Geometry: final body of the model. Coordinates: model frame, mm. Face numbers are marked on the shaded views. A direction names the side the tool comes from. Give positions to 0.01 mm unless a question says otherwise; leave off trailing zeros. Loops run counter-clockwise (first coordinate to the right, second up) from the corner with the lowest first, then second, coordinate; pieces in that order, holes last. Notation, with made-up numbers: (47, 11) - (105, 11) arc R22 cw to (105, 39) - close; hole circle Ø1 at (37.25, 12). An arc over 180 degrees is marked (long way). Answer in a Markdown table with one row per item.
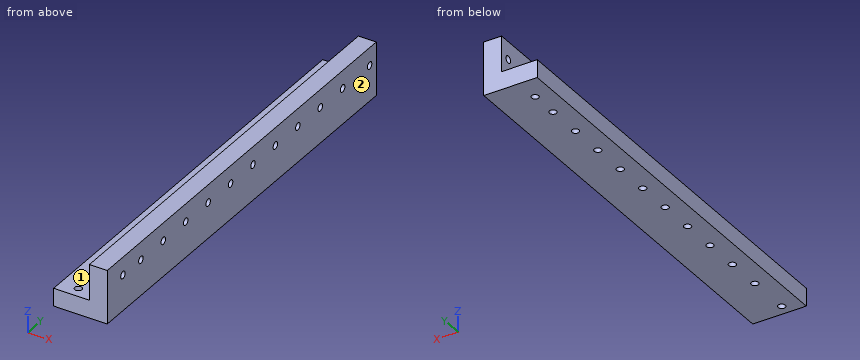
from build123d import *

# Parameters (mm, degrees)
BOSS_EXTRUDE1_DEPTH = 120
SKETCH2_R           = 1
CUT_EXTRUDE3_DEPTH  = 120
SKETCH4_R           = 1
CUT_EXTRUDE4_DEPTH  = 120
SKETCH5_R           = 1
CUT_EXTRUDE5_DEPTH  = 120
SKETCH6_R           = 1
CUT_EXTRUDE6_DEPTH  = 120
SKETCH8_R           = 1
CUT_EXTRUDE7_DEPTH  = 120
SKETCH9_R           = 1
CUT_EXTRUDE8_DEPTH  = 120


with BuildPart() as part:
    # Sketch1 → Boss-Extrude1 (new body)
    with BuildSketch(Plane(origin=(0, 0, 0), x_dir=(1, 0, 0), z_dir=(0, 1, 0))):
        Polygon((-19.661478752, 6.607142857), (-4.661478752, 6.607142857), (-4.661478752, -8.392857143), (-9.661478752, -8.392857143), (-9.661478752, 1.607142857), (-19.661478752, 1.607142857), align=None)
    extrude(amount=BOSS_EXTRUDE1_DEPTH)

    # Sketch2 → Cut-Extrude3 (cut)
    with BuildSketch(Plane(origin=(-4.661478752, 0, 0), x_dir=(0, 0, -1), z_dir=(1, 0, 0))):
        with Locations((-3.392857143, 117)):
            Circle(SKETCH2_R)
    extrude(amount=-CUT_EXTRUDE3_DEPTH, mode=Mode.SUBTRACT)

    # Sketch4 → Cut-Extrude4 (cut)
    with BuildSketch(Plane(origin=(0, 0, -6.607142857), x_dir=(-1, 0, 0), z_dir=(0, 0, -1))):
        with Locations((14.661478752, 113)):
            Circle(SKETCH4_R)
    extrude(amount=-CUT_EXTRUDE4_DEPTH, mode=Mode.SUBTRACT)

    # Sketch5 → Cut-Extrude5 (cut)
    with BuildSketch(Plane(origin=(-4.661478752, 0, 0), x_dir=(0, 0, -1), z_dir=(1, 0, 0))):
        with Locations((-3.392857143, 7)):
            Circle(SKETCH5_R)
    extrude(amount=-CUT_EXTRUDE5_DEPTH, mode=Mode.SUBTRACT)

    # Sketch6 → Cut-Extrude6 (cut)
    with BuildSketch(Plane(origin=(0, 0, -6.607142857), x_dir=(-1, 0, 0), z_dir=(0, 0, -1))):
        with Locations((14.661478752, 3)):
            Circle(SKETCH6_R)
    extrude(amount=-CUT_EXTRUDE6_DEPTH, mode=Mode.SUBTRACT)

    # Sketch8 → Cut-Extrude7 (cut)
    with BuildSketch(Plane(origin=(-4.661478752, 0, 0), x_dir=(0, 0, -1), z_dir=(1, 0, 0))):
        with Locations((-3.392857143, 105)):
            Circle(SKETCH8_R)
        with Locations((-3.392857143, 95)):
            Circle(SKETCH8_R)
        with Locations((-3.392857143, 85)):
            Circle(SKETCH8_R)
        with Locations((-3.392857143, 75)):
            Circle(SKETCH8_R)
        with Locations((-3.392857143, 65)):
            Circle(SKETCH8_R)
        with Locations((-3.392857143, 55)):
            Circle(SKETCH8_R)
        with Locations((-3.392857143, 45)):
            Circle(SKETCH8_R)
        with Locations((-3.392857143, 35)):
            Circle(SKETCH8_R)
        with Locations((-3.392857143, 25)):
            Circle(SKETCH8_R)
        with Locations((-3.392857143, 15)):
            Circle(SKETCH8_R)
    extrude(amount=-CUT_EXTRUDE7_DEPTH, mode=Mode.SUBTRACT)

    # Sketch9 → Cut-Extrude8 (cut)
    with BuildSketch(Plane(origin=(0, 0, -6.607142857), x_dir=(-1, 0, 0), z_dir=(0, 0, -1))):
        with Locations((14.661478752, 15)):
            Circle(SKETCH9_R)
        with Locations((14.661478752, 25)):
            Circle(SKETCH9_R)
        with Locations((14.661478752, 35)):
            Circle(SKETCH9_R)
        with Locations((14.661478752, 45)):
            Circle(SKETCH9_R)
        with Locations((14.661478752, 55)):
            Circle(SKETCH9_R)
        with Locations((14.661478752, 65)):
            Circle(SKETCH9_R)
        with Locations((14.661478752, 75)):
            Circle(SKETCH9_R)
        with Locations((14.661478752, 85)):
            Circle(SKETCH9_R)
        with Locations((14.661478752, 95)):
            Circle(SKETCH9_R)
        with Locations((14.661478752, 105)):
            Circle(SKETCH9_R)
    extrude(amount=-CUT_EXTRUDE8_DEPTH, mode=Mode.SUBTRACT)


solid = part.part
Q1. Reachability of the marked faces 1 and 2 from +Z, -Z, +X, -X, +Y, -Y: full face, straight path, thin tool, end or side. Return the list, or none.
Check values:
| item | result |
|---|---|
| face 1 | +Z, -X, +Y, -Y |
| face 2 | +Z, -Z, +X, +Y, -Y |
Q2. Cut plane A-A (y = 65). Output: boundary loops of the cut face in (x, z), and give its area (3 significant figures).
Check values:
| item | result |
|---|---|
| outline | (-19.66, -6.61) - (-15.66, -6.61) - (-15.66, -1.61) - (-19.66, -1.61) - close; (-13.66, -6.61) - (-4.66, -6.61) - (-4.66, 2.39) - (-9.66, 2.39) - (-9.66, -1.61) - (-13.66, -1.61) - close; (-9.66, 4.39) - (-4.66, 4.39) - (-4.66, 8.39) - (-9.66, 8.39) - close |
| area | 105 mm² |
Q3. Material intervals for line 1 along Z through (x, y) = (-6.15, 105); line 2 along Z through (x, y) = (-12.5, 10.5); line 3 along X through (y, z) = (113, -4.45), sorted ascending.
Check values:
| item | result |
|---|---|
| line 1 | -6.61 to 2.39, 4.39 to 8.39 |
| line 2 | -6.61 to -1.61 |
| line 3 | -19.66 to -15.66, -13.66 to -4.66 |
Q4. Cut plane B-B (z = -3.25). Give the number of separate pieces and of enclosed holes in the cut face, and give its area (3 significant figures).
Check values:
| item | result |
|---|---|
| separate pieces | 1 |
| enclosed holes | 12 |
| area | 1,760 mm² |
Q5. First-contact query: pin 1 (3 mm diameter, centred on y = 7, z = 3.39, fed in from -X); pin 2 (3 mm diameter, centred on x = -14.66, y = 25, fed in from +Z); pin 3 (1.6 mm diameter, centred on y = 75, z = 3.39, fed in from +X). Flat tips, straight axial feed; report the tip coordinate or a pass-through.
Check values:
| item | result |
|---|---|
| pin 1 | x = -9.66 |
| pin 2 | z = -1.61 |
| pin 3 | through |
Q6. Cut plane D-D (z = 5.75). Output: boundary loops of the cut face in (x, y).
Check values:
| item | result |
|---|---|
| outline | (-9.66, 0) - (-4.66, 0) - (-4.66, 120) - (-9.66, 120) - close |
Q7. Cut plane C-C (y = 113). Output: boundary loops of the cut face in (x, z).
Check values:
| item | result |
|---|---|
| outline | (-19.66, -6.61) - (-15.66, -6.61) - (-15.66, -1.61) - (-19.66, -1.61) - close; (-13.66, -6.61) - (-4.66, -6.61) - (-4.66, 8.39) - (-9.66, 8.39) - (-9.66, -1.61) - (-13.66, -1.61) - close |
